Design review of the part built by this model. Coordinates are the model's own, in mm. A direction names the side the tool comes from. Round coordinates to 2 decimals unless told otherwise and drop trailing zeros. Loops run counter-clockwise (first coordinate to the right, second up) from the corner with the lowest first, then second, coordinate; pieces in that order, holes last. Notation, with made-up numbers: (-4.75, -0.75) - (26.25, -0.75) arc R20 ccw to (26.25, 21.25) - close; hole circle Ø4 at (82, 2). An arc over 180 degrees is marked (long way). Return JSON: item names as keys, results as strings. Group by question number.
(1) The part is to be moulded in two halves that separate along Z. For faces 4 (the cylindrical face through (0, -7, -6)), 5 (the flat face through (0, -10.2, -13)), 6 (the cylindrical face through (-2.799, -3.986, 21.317)), say which applies: pulls with the +Z half, pulls with the -Z half, needs draft (parallel to the pull), parting line crosses it, or undercut.
(2) We need section D-D, the plane x = 7.5. Write out the cut boundary in (y, z).
(3) Clearance check with flat-ended pins moving along their axes: pin 1 (12 mm diameter, centred on x = 0, z = -4.5, fed in from -Y); pin 2 (1 mm diameter, centred on y = -9, z = 10.5, fed in from +X); pin 3 (2 mm diameter, centred on x = -14.5, z = 8, fed in from -Y). State where each tip first meets the part, or that it passes through.
(4) We need section B-B, the plane x = 0. Write out the cut boundary in (y, z).
(5) We need section A-A, the plane z = 0. Write out the cut boundary in (x, y), and give its area (3 significant figures).
(6) For faces 1 (the cylindrical face through (0, -7, -16)), 2 (the flat face through (0, -7, 7.641)), 3 (the flat face through (14, -10.2, 14)), list the 3-axis set-ups (+Z, -Z, +X, -X, +Y, -Y) from which the entire face can be reached by the end or side of a thin tool; tool diameter is ignored.
(7) We need section C-C, the plane y = -4.5. Write out the cut boundary in (x, z), and give its area (3 significant figures).
(8) Wall thickness on L1, parallel to X at y = -7.5, z = 0; L2, parallel to X at y = -6.25, z = -5.5; L3, parallel to Y at x = -5, z = -17: over which ranges is each line inside the solid? List them lowest first. Write a range as [from, to].
from build123d import *

# Parameters (mm, degrees)
SKETCH_R        = 21.5
PAD_DEPTH       = 2
SKETCH031_R     = 1.5
PAD015_DEPTH    = 5.2
PAD016_DEPTH    = 4.2
SKETCH032_R     = 1.5
PAD017_DEPTH    = 1
POCKET018_DEPTH = 4
SKETCH036_R     = 3
POCKET019_DEPTH = 7.201
SKETCH038_R     = 3
POCKET022_DEPTH = 7.201


with BuildPart() as part:
    # Sketch → Pad (new body)
    with BuildSketch(Plane.XZ):
        Circle(SKETCH_R)
    extrude(amount=PAD_DEPTH)

    # Sketch031 (on Face3 of Pad) → Pad015 (join)
    with BuildSketch(Plane.XZ.offset(2)):
        with Locations((-14.142136, 14.142136)):
            Circle(SKETCH031_R)
        with Locations((14.142136, 14.142136)):
            Circle(SKETCH031_R)
    extrude(amount=PAD015_DEPTH)

    # Sketch017 (on Face3 of Pad) → Pad016 (join)
    with BuildSketch(Plane.XZ.offset(2)):
        with BuildLine():
            ThreePointArc((-15.403137, 4.329363), (-8.931504, 4.97358), (-3, 7.640846))
            Line((-3, 7.640846), (3, 7.640846))
            ThreePointArc((3, 7.640846), (8.931504, 4.97358), (15.403137, 4.329363))
            ThreePointArc((-15.403137, 4.329363), (0, -16), (15.403137, 4.329363))
        make_face()
    extrude(amount=PAD016_DEPTH)

    # Sketch032 (on Face11 of Pad016) → Pad017 (join)
    with BuildSketch(Plane.XZ.offset(6.2)):
        with Locations((0, -13.5)):
            Circle(SKETCH032_R)
    extrude(amount=PAD017_DEPTH)

    # Sketch035 (on Face11 of Pad017) → Pocket018 (cut)
    with BuildSketch(Plane.XZ.offset(6.2)):
        with BuildLine():
            ThreePointArc((-12.932656, 1.321513), (-8.953461, 1.877631), (-5.129887, 3.111954))
            ThreePointArc((-5.129887, 3.111954), (0, -6), (5.129887, 3.111954))
            ThreePointArc((5.129887, 3.111954), (8.953461, 1.877631), (12.932656, 1.321513))
            ThreePointArc((2.884597, -12.675926), (10.560703, -7.580999), (12.932656, 1.321513))
            ThreePointArc((2.884597, -12.675926), (0, -10.5), (-2.884597, -12.675926))
            ThreePointArc((-12.932656, 1.321513), (-10.560703, -7.580999), (-2.884597, -12.675926))
        make_face()
    extrude(amount=-POCKET018_DEPTH, mode=Mode.SUBTRACT)

    # Sketch036 (on Face2 of Pocket018) → Pocket019 (cut, through all)
    with BuildSketch(Plane(origin=(0, 0, 0), x_dir=(1, 0, 0), z_dir=(0, 1, 0))):
        Circle(SKETCH036_R)
    extrude(amount=-POCKET019_DEPTH, mode=Mode.SUBTRACT)

    # Sketch038 (on Face2 of Pad016) → Pocket022 (cut, through all)
    with BuildSketch(Plane(origin=(0, 0, 0), x_dir=(1, 0, 0), z_dir=(0, 1, 0))):
        Circle(SKETCH038_R)
    extrude(amount=-POCKET022_DEPTH, mode=Mode.SUBTRACT)


with BuildPart() as part_1:
    # Body placement: moved
    add(part.part.moved(Location((0, -3, 0))))


solid = part_1.part
Solutions:
{
 "1": {"face 4": "undercut", "face 5": "needs draft", "face 6": "parting line crosses it"},
 "2": {"outline": "(-9.2, -14.13) - (-5, -14.13) - (-5, -20.15) - (-3, -20.15) - (-3, 20.15) - (-5, 20.15) - (-5, 5.41) - (-9.2, 5.41) - (-9.2, 2.26) - (-5.2, 2.26) - (-5.2, -10.62) - (-9.2, -10.62) - close"},
 "3": {"pin 1": "y = -9.2", "pin 2": "through", "pin 3": "y = -5"},
 "4": {"outline": "(-10.2, -15) - (-9.2, -15) - (-9.2, -16) - (-5, -16) - (-5, -21.5) - (-3, -21.5) - (-3, -3) - (-9.2, -3) - (-9.2, -6) - (-5.2, -6) - (-5.2, -10.5) - (-9.2, -10.5) - (-9.2, -12) - (-10.2, -12) - close; (-9.2, 3) - (-3, 3) - (-3, 21.5) - (-5, 21.5) - (-5, 7.64) - (-9.2, 7.64) - close"},
 "5": {"outline": "(-21.5, -5) - (-16, -5) - (-16, -9.2) - (-13, -9.2) - (-13, -5.2) - (-6, -5.2) - (-6, -9.2) - (-3, -9.2) - (-3, -3) - (-21.5, -3) - close; (3, -9.2) - (6, -9.2) - (6, -5.2) - (13, -5.2) - (13, -9.2) - (16, -9.2) - (16, -5) - (21.5, -5) - (21.5, -3) - (3, -3) - close", "area": "127 mm^2"},
 "6": {"face 1": "-Y", "face 2": "+Z, +X, -X, -Y", "face 3": "+Z, -Z, +X, -X, -Y"},
 "7": {"outline": "circle Ø43 at (0, 0); hole circle Ø6 at (0, 0)", "area": "1,420 mm^2"},
 "8": {"L1": "[-16, -13], [-6, -3], [3, 6], [13, 16]", "L2": "[-15.02, -11.78], [-2.4, 2.4], [11.78, 15.02]", "L3": "[-5, -3]"}
}
